from build123d import *

# Parameters (mm, degrees)
F2_SIZE = 1.5
F3_SIZE = 1.5


with BuildPart() as f1:
    # F0 (on Front) → F1 (revolve)
    with BuildSketch(Plane.XZ):
        with BuildLine():
            Line((5, 13.1), (5, 13.038275))
            ThreePointArc((5, 13.038275), (4.12132, 10.916955), (2, 10.038275))
            Line((2, 10.038275), (-115, 10.038275))
            Line((-115, 10.038275), (-115, 0))
            Line((-115, 0), (56.999728, 0))
            Line((56.999728, 0), (56.999728, 9))
            Line((56.999728, 9), (31.999728, 9))
            Line((31.999728, 9), (30.143602, 7.910138))
            Line((30.143602, 7.910138), (27.029878, 7.910138))
            Line((27.029878, 7.910138), (25.173751, 9))
            Line((25.173751, 9), (12.615061, 9))
            ThreePointArc((12.615061, 9), (12.179955, 9.180227), (11.999728, 9.615333))
            Line((11.999728, 9.615333), (11.999728, 13.038275))
            Line((11.999728, 13.038275), (5, 13.1))
        make_face()
    revolve(axis=Axis((-29.000136, 0, 0), (1, 0, 0)))

    # F2
    f2_edges = [f1.edges().sort_by_distance(p)[0] for p in [
        (56.999728, 0, -9),
    ]]
    chamfer(f2_edges, length=F2_SIZE)

    # F3
    f3_edges = [f1.edges().sort_by_distance(p)[0] for p in [
        (-115, 0, -10.038275),
    ]]
    chamfer(f3_edges, length=F3_SIZE)


solid = f1.part
CAD build for the part. Positions are in the model's coordinates, mm. A direction names the side the tool comes from. Coordinates: 2 decimals unless noted, no trailing zeros. Loops run counter-clockwise (first coordinate to the right, second up) from the corner with the lowest first, then second, coordinate; pieces in that order, holes last. Notation, with made-up numbers: (21, 10.5) - (45, 10.5) arc R21 ccw to (45, 16.5) - close; hole circle Ø4 at (22.25, 62.5). An arc over 180 degrees is marked (long way). Use one line per item in the form item = value. Start each with the question number.
1) Flat gauge pins, fed straight in: pin 1 (5 mm diameter, centred on x = -3, z = 1, fed in from -Y); pin 2 (8 mm diameter, centred on x = -85, y = 2, fed in from +Z); pin 3 (10 mm diameter, centred on x = 16, z = 2.5, fed in from +Y). Where does each tip first touch, or does it go through?
2) Drill centre lines: L1, parallel to Y at x = -10.5, z = -0.25; L2, parallel to Y at x = -6, z = -4.5; L3, parallel to X at y = -2.75, z = 8. Where is each one in solid material? Low to high. Write a range as from..to.
3) Band-saw the part on B-B (x = 3.5). Give the cut face in (y, z).
4) Two-plate mould, pull along X, no slides. Class faces 1 (the face through (8.451, -0.575, -13.057)), 2 (the face through (28.565, 7.722, -1.715)), 3 (the face through (43.585, -8.923, -1.172)): +X half, -X half, draft (parallel to the pull), parting line (faces both ways), or undercut.
5) Tool access for faces 4 (the face through (-56.56, 9.8, -2.18)), 5 (the face through (12, 10, 1)), 6 (the face through (-115, 0, 0)): list every direction of +Z, -Z, +X, -X, +Y, -Y with a clear straight run to the whole face (end or side of a thin tool).
6) Band-saw the part on A-A (x = -29.5). Give the cut face in (y, z).
Check values:
q1.pin_1 = -10.04
q1.pin_2 = 10.04
q1.pin_3 = 13.04
q2.L1 = -10.04..10.04
q2.L2 = -8.97..8.97
q2.L3 = -115..26.09, 31.08..56.04
q3.outline = circle Ø20.88 at (0, 0)
q4.face_1 = +X half
q4.face_2 = undercut
q4.face_3 = draft
q5.face_4 = -X
q5.face_5 = +X
q5.face_6 = +Z, -Z, -X, +Y, -Y
q6.outline = circle Ø20.08 at (0, 0)
